Input: part model. Units: mm. Frame: model coordinates. A direction names the side the tool comes from. Round coordinates to 2 decimals unless told otherwise and drop trailing zeros. Loops run counter-clockwise (first coordinate to the right, second up) from the corner with the lowest first, then second, coordinate; pieces in that order, holes last. Notation, with made-up numbers: (44, 7) -> (74, 7) arc R19 cw to (74, 29) -> close; hole circle Ø2 at (4, -5.75). An arc over 180 degrees is marked (long way). Answer as a JSON object with one key per item and string values.
```python
from build123d import *

# Parameters (mm, degrees)
EXTRUDE_1_DEPTH     = 3
SKETCH_2_R          = 1.6
SKETCH_2_R_2        = 12
CUT_EXTRUDE_1_DEPTH = 3
SKETCH_4_R          = 1.625
CUT_EXTRUDE_2_DEPTH = 96.765338197


with BuildPart() as part:
    # 草图1 → 凸台-拉伸1 (new body)
    with BuildSketch(Plane(origin=(0, 0, 0), x_dir=(1, 0, 0), z_dir=(0, 1, 0))):
        Polygon((0, 0), (0, 36), (35, 36), (35, 51), (81, 51), (81, -15), (35, -15), (35, 0), align=None)
    extrude(amount=EXTRUDE_1_DEPTH)

    # 草图2 → 切除-拉伸1 (cut)
    with BuildSketch(Plane(origin=(0, 3, 0), x_dir=(1, 0, 0), z_dir=(0, 1, 0))):
        with Locations(Location((8, 28, 0), (0, 0, 270))):
            Circle(SKETCH_2_R)
        with Locations(Location((23, 28, 0), (0, 0, 270))):
            Circle(SKETCH_2_R)
        with Locations(Location((8, 8, 0), (0, 0, 270))):
            Circle(SKETCH_2_R)
        with Locations(Location((23, 8, 0), (0, 0, 270))):
            Circle(SKETCH_2_R)
        with Locations(Location((61, 18, 0), (0, 0, 270))):
            Circle(SKETCH_2_R_2)
    extrude(amount=-CUT_EXTRUDE_1_DEPTH, mode=Mode.SUBTRACT)

    # 草图4 → 切除-拉伸2 (cut, through all)
    with BuildSketch(Plane.XZ):
        with Locations(Location((45.5, -33.5, 0), (0, 0, 270))):
            Circle(SKETCH_4_R)
        with Locations(Location((76.5, -33.5, 0), (0, 0, 270))):
            Circle(SKETCH_4_R)
        with Locations(Location((76.5, -2.5, 0), (0, 0, 270))):
            Circle(SKETCH_4_R)
        with Locations(Location((45.5, -2.5, 0), (0, 0, 270))):
            Circle(SKETCH_4_R)
    extrude(amount=-CUT_EXTRUDE_2_DEPTH, mode=Mode.SUBTRACT)


solid = part.part
```
1) Section C-C, the plane x = 61. Output: boundary loops of the cut face in (y, z).
Output:
{"outline": "(0, -51) -> (3, -51) -> (3, -30) -> (0, -30) -> close; (0, -6) -> (3, -6) -> (3, 15) -> (0, 15) -> close"}
2) Section B-B, the plane z = -28. Output: boundary loops of the cut face in (x, y).
Output:
{"outline": "(0, 0) -> (6.4, 0) -> (6.4, 3) -> (0, 3) -> close; (9.6, 0) -> (21.4, 0) -> (21.4, 3) -> (9.6, 3) -> close; (24.6, 0) -> (54.37, 0) -> (54.37, 3) -> (24.6, 3) -> close; (67.63, 0) -> (81, 0) -> (81, 3) -> (67.63, 3) -> close"}
3) Draft query along X for faces 4 (the face through (41, 3, -18)), 5 (the face through (7.03, 1.52, -29.27)), 6 (the face through (0, 1, -18)). Return one class per face: +X half, -X half, draft (parallel to the pull), parting line (faces both ways), or undercut.
Output:
{"face 4": "draft", "face 5": "undercut", "face 6": "-X half"}
4) Section D-D, the plane y = 1.8. Count the separate pieces of the cut face and the enclosed holes in it, plus the area to 3 significant figures.
Output:
{"separate pieces": "1", "enclosed holes": "9", "area": "3,780 mm^2"}
5) Section A-A, the plane x = 23. Output: boundary loops of the cut face in (y, z), plus the area to 3 significant figures.
Output:
{"outline": "(0, -36) -> (3, -36) -> (3, -29.6) -> (0, -29.6) -> close; (0, -26.4) -> (3, -26.4) -> (3, -9.6) -> (0, -9.6) -> close; (0, -6.4) -> (3, -6.4) -> (3, 0) -> (0, 0) -> close", "area": "88.8 mm^2"}
6) Reachability of faces 1 (the face through (43.914, 1.479, -2.148)), 2 (the face through (17, 1, -36)), 3 (the face through (18, 1, 0)) from +Z, -Z, +X, -X, +Y, -Y: full face, straight path, thin tool, end or side. Return the list, or none.
Output:
{"face 1": "+Y, -Y", "face 2": "-Z, -X, +Y, -Y", "face 3": "+Z, -X, +Y, -Y"}
7) Contact query for flat-ended pins moving along their axis: P1, Ø1.9, axis at x = 76.5, z = -33.5, coming from the +Y side; P2, Ø8, axis at x = 48.5, z = -25, coming from the -Y side. Output: stop coordinate, or through.
Output:
{"P1": "passes through", "P2": "stops at y = 0"}
8) Ray query, probe 1 along Z at (x, y) = (76.5, 0.85) (3 decimals); probe 2 along X at (y, z) = (1.7, -2.5) (3 decimals); probe 3 along X at (y, z) = (2, -18). Return the intervals inside material, ascending.
Output:
{"probe 1": "z = -51 to -35.125, -31.875 to -4.125, -0.875 to 15", "probe 2": "x = 0 to 43.875, 47.125 to 74.875, 78.125 to 81", "probe 3": "x = 0 to 49, 73 to 81"}
